```python
from build123d import *

# Parameters (mm, degrees)
F0_W     = 114.3
F0_H     = 63.5
F1_DEPTH = 3.1242


with BuildPart() as f1:
    # F0 (on Front) → F1 (new body)
    with BuildSketch(Plane.XZ):
        with Locations((39.126127, 17.265163)):
            Rectangle(F0_W, F0_H)
        with BuildLine():
            ThreePointArc((46.28682, -2.245064), (41.796692, -2.245064), (41.796692, 2.245064))
            Line((41.796692, 2.245064), (56.816791, 17.265163))
            Line((56.816791, 17.265163), (41.796692, 32.285263))
            ThreePointArc((41.796692, 32.285263), (41.796692, 36.775391), (46.28682, 36.775391))
            Line((46.28682, 36.775391), (63.551983, 19.510227))
            ThreePointArc((63.551983, 19.510227), (64.481919, 17.265163), (63.551983, 15.020099))
            Line((63.551983, 15.020099), (46.28682, -2.245064))
        make_face(mode=Mode.SUBTRACT)
        with BuildLine():
            ThreePointArc((74.762899, 0), (71.587899, -3.175), (68.412899, 0))
            Line((68.412899, 0), (68.412899, 17.265163))
            Line((68.412899, 17.265163), (68.412899, 34.530327))
            ThreePointArc((68.412899, 34.530327), (71.587899, 37.705327), (74.762899, 34.530327))
            Line((74.762899, 34.530327), (74.762899, 17.265163))
            Line((74.762899, 17.265163), (74.762899, 0))
        make_face(mode=Mode.SUBTRACT)
        with BuildLine():
            ThreePointArc((2.877527, -1.341813), (-1.341813, -2.877527), (-2.877527, 1.341813))
            Line((-2.877527, 1.341813), (13.224229, 35.87214))
            ThreePointArc((13.224229, 35.87214), (16.101756, 37.705327), (18.979283, 35.87214))
            Line((18.979283, 35.87214), (35.081039, 1.341813))
            ThreePointArc((35.081039, 1.341813), (33.545325, -2.877527), (29.325984, -1.341813))
            Line((29.325984, -1.341813), (16.101756, 27.017637))
            Line((16.101756, 27.017637), (2.877527, -1.341813))
        make_face(mode=Mode.SUBTRACT)
    extrude(amount=F1_DEPTH)


solid = f1.part
```
The listing builds one solid part. Answer for the finished solid, in the listing's coordinates (mm). A direction names the side the tool comes from. Coordinates: 2 decimals unless noted, no trailing zeros. Loops run counter-clockwise (first coordinate to the right, second up) from the corner with the lowest first, then second, coordinate; pieces in that order, holes last. Notation, with made-up numbers: (45, 24) -> (58, 24) arc R14 ccw to (58, 51) -> close; hole circle Ø3 at (47.25, 46.25). An arc over 180 degrees is marked (long way). Return JSON: item names as keys, results as strings. Group by question number.
(1) Find the intervals of material crossed by probe 1 along Z at (x, y) = (56, -0.9); probe 2 along X at (y, z) = (-0.4, 30.5); probe 3 along Z at (x, y) = (46, -2.45), in increasing order. Write a range as from..to.
(2) Determine the mould class of faces 3 (the flat face through (96.276, -2, 17)), 4 (the flat face through (-18.024, -2, 17)), 5 (the cylindrical face through (16.051, -1.54, 37.705)) for opening direction X: released by +X, released by -X, zero draft, split by the parting line, or undercut.
(3) A cutting plane is placed at C-C on z = 11. Write down the section's boundary in (x, y).
(4) Which of the six approach directions +Z, -Z, +X, -X, +Y, -Y give full straight-line access (tool end or side, diameter ignored) to faces 1 (the flat face through (54.8, -1.54, 28.26)), 2 (the flat face through (38, -3.124, 18))?
(5) A cutting plane is placed at B-B on x = 0. Write down the section's boundary in (y, z) (3 decimals), and give its area (3 significant figures).
(6) A cutting plane is placed at A-A on y = -1.95. Write down the section's boundary in (x, z) (3 decimals), and give its area (3 significant figures).
(7) A cutting plane is placed at D-D on x = 50. Write down the section's boundary in (y, z), and give its area (3 significant figures).
The answers:
{
 "1": {"probe 1": "z = -14.48..7.47, 16.45..18.08, 27.06..49.02", "probe 2": "x = -18.02..10.72, 21.48..43.58, 52.56..68.41, 74.76..96.28", "probe 3": "z = -14.48..-2.5, 6.45..28.08, 37.03..49.02"},
 "2": {"face 3": "released by +X", "face 4": "released by -X", "face 5": "undercut"},
 "3": {"outline": "(-18.02, -3.12) -> (1.63, -3.12) -> (1.63, 0) -> (-18.02, 0) -> close; (8.63, -3.12) -> (23.57, -3.12) -> (23.57, 0) -> (8.63, 0) -> close; (30.58, -3.12) -> (50.55, -3.12) -> (50.55, 0) -> (30.58, 0) -> close; (59.53, -3.12) -> (68.41, -3.12) -> (68.41, 0) -> (59.53, 0) -> close; (74.76, -3.12) -> (96.28, -3.12) -> (96.28, 0) -> (74.76, 0) -> close"},
 "4": {"face 1": "+Y, -Y", "face 2": "+Z, -Z, +X, -X, -Y"},
 "5": {"outline": "(-3.124, -14.485) -> (0, -14.485) -> (0, -3.175) -> (-3.124, -3.175) -> close; (-3.124, 7.513) -> (0, 7.513) -> (0, 49.015) -> (-3.124, 49.015) -> close", "area": "165 mm^2"},
 "6": {"outline": "(-18.024, -14.485) -> (96.276, -14.485) -> (96.276, 49.015) -> (-18.024, 49.015) -> close; hole (-2.878, 1.342) arc R3.175 ccw to (2.878, -1.342) -> (16.102, 27.018) -> (29.326, -1.342) arc R3.175 ccw to (35.081, 1.342) -> (18.979, 35.872) arc R3.175 ccw to (13.224, 35.872) -> close; hole (41.797, 2.245) arc R3.175 ccw to (46.287, -2.245) -> (63.552, 15.02) arc R3.175 ccw to (63.552, 19.51) -> (46.287, 36.775) arc R3.175 ccw to (41.797, 32.285) -> (56.817, 17.265) -> close; hole (68.413, 0) arc R3.175 ccw to (74.763, 0) -> (74.763, 34.53) arc R3.175 ccw to (68.413, 34.53) -> close", "area": "6,160 mm^2"},
 "7": {"outline": "(-3.12, -14.48) -> (0, -14.48) -> (0, 1.47) -> (-3.12, 1.47) -> close; (-3.12, 10.45) -> (0, 10.45) -> (0, 24.08) -> (-3.12, 24.08) -> close; (-3.12, 33.06) -> (0, 33.06) -> (0, 49.02) -> (-3.12, 49.02) -> close", "area": "142 mm^2"}
}
